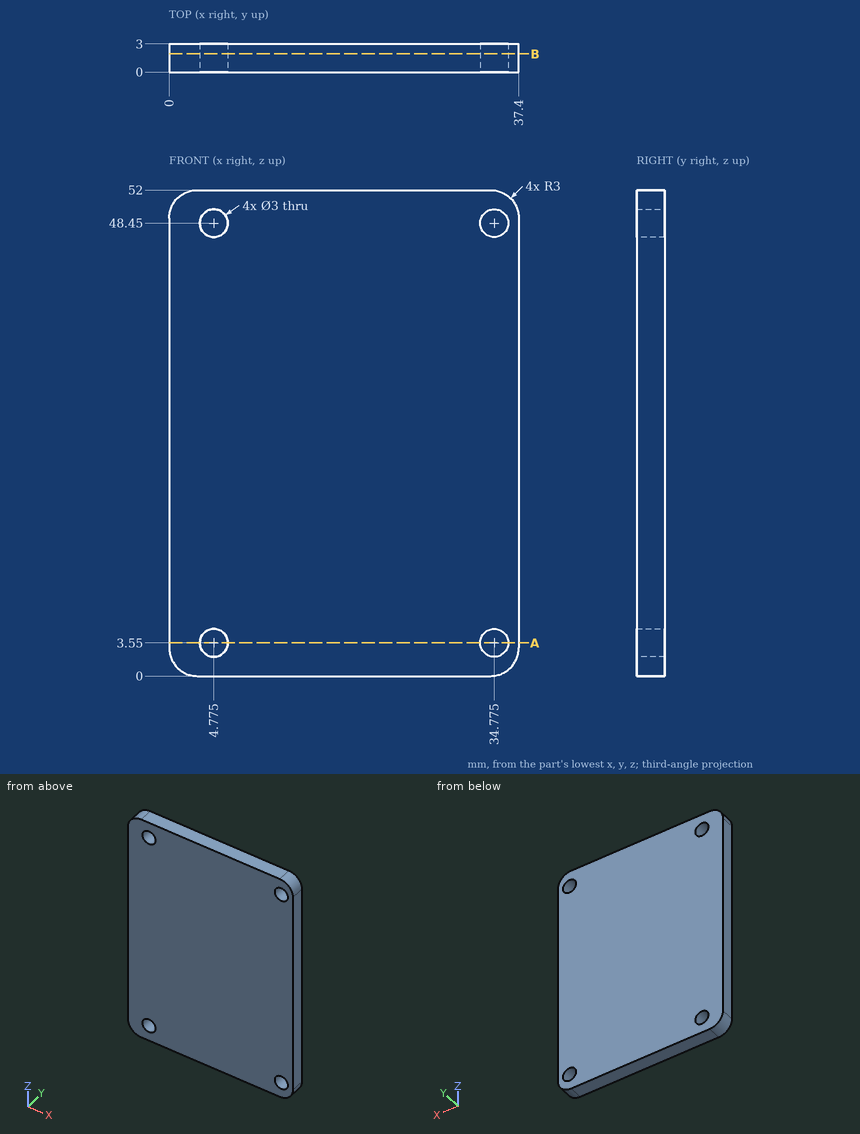
Print and shaded views of the part. All mm, measured from the part's lowest x, y and z. Round coordinates to 2 decimals unless told otherwise and drop trailing zeros. Write each loop counter-clockwise with the first axis right and the second up, starting at its lowest first coordinate (ties: lowest second). Pieces come first, ordered by that corner, then holes. Notation, with made-up numbers: (45, -33.5) - (88, -33.5) arc R33 ccw to (88, -2.5) - close; hole circle Ø4 at (-32.75, 86). An arc over 180 degrees is marked (long way). Write each question's results on one line, items separated by ' | '. Start each with the question number.
Item 1: Saw through at A-A (z = 3.55). Write the cut outline in (x, y) (3 decimals).
Item 2: Wall check: L1, parallel to X at y = 2.05, z = 48.45 (3 decimals); L2, parallel to X at y = 0.5, z = 4.5; L3, parallel to Z at x = 33.5, y = 1.65. Give the ranges that are in metal, low to high. Write a range as [from, to].
Item 3: Saw through at B-B (y = 1.95). Write the cut outline in (x, z) (3 decimals).
Results are:
1) outline: (0, 0) - (3.275, 0) - (3.275, 3) - (0, 3) - close; (6.275, 0) - (33.275, 0) - (33.275, 3) - (6.275, 3) - close; (36.275, 0) - (37.4, 0) - (37.4, 3) - (36.275, 3) - close
2) L1: x = [0, 3.275], [6.275, 33.275], [36.275, 37.4] | L2: x = [0, 3.61], [5.94, 33.61], [35.94, 37.4] | L3: z = [0, 2.76], [4.34, 47.66], [49.24, 52]
3) outline: (0, 3) arc R3 ccw to (3, 0) - (34.4, 0) arc R3 ccw to (37.4, 3) - (37.4, 49) arc R3 ccw to (34.4, 52) - (3, 52) arc R3 ccw to (0, 49) - close; hole circle Ø3 at (4.775, 3.55); hole circle Ø3 at (4.775, 48.45); hole circle Ø3 at (34.775, 3.55); hole circle Ø3 at (34.775, 48.45)
